```python
from build123d import *

# Parameters (mm, degrees)
BOSS_EXTRUDE1_DEPTH = 6.35
SKETCH2_R           = 2.5
CUT_EXTRUDE1_DEPTH  = 103.686827993


with BuildPart() as part:
    # Sketch1 → Boss-Extrude1 (new body)
    with BuildSketch(Plane(origin=(0, 0, 0), x_dir=(1, 0, 0), z_dir=(0, 1, 0))):
        with BuildLine():
            Line((5.368406408, 0), (44.345824206, 0))
            ThreePointArc((44.345824206, 0), (46.333684351, 0.753132838), (47.323462661, 2.63439197))
            Line((47.323462661, 2.63439197), (57.040137924, 81.77036144))
            ThreePointArc((57.040137924, 81.77036144), (55.05416359, 84.967329968), (51.507452969, 83.708145472))
            Line((51.507452969, 83.708145472), (2.813359907, 4.572176002))
            ThreePointArc((2.813359907, 4.572176002), (2.749577661, 1.536532885), (5.368406408, 0))
        make_face()
    extrude(amount=BOSS_EXTRUDE1_DEPTH)

    # Sketch2 → Cut-Extrude1 (cut, through all)
    with BuildSketch(Plane(origin=(0, 6.35, 0), x_dir=(1, 0, 0), z_dir=(0, 1, 0))):
        with Locations(Location((13.421016019, 7.5, 0), (0, 0, 270))):
            Circle(SKETCH2_R)
        with Locations(Location((46.29547273, 60.926439205, 0), (0, 0, 270))):
            Circle(SKETCH2_R)
        with Locations(Location((39.735530851, 7.5, 0), (0, 0, 270))):
            Circle(SKETCH2_R)
    extrude(amount=-CUT_EXTRUDE1_DEPTH, mode=Mode.SUBTRACT)


solid = part.part
```
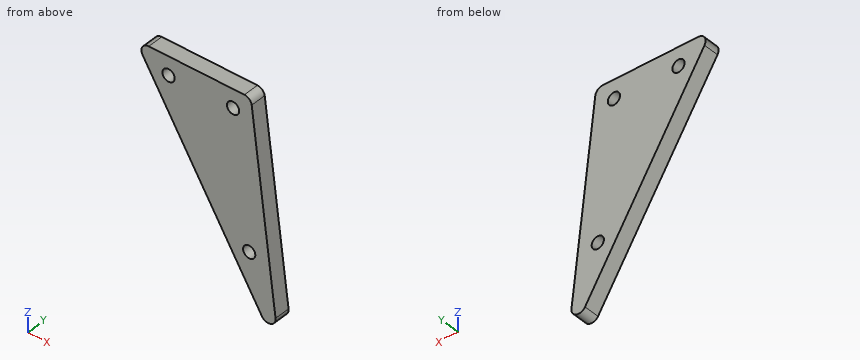
Design review of the part built by this model. Coordinates are the model's own, in mm. Give positions to 0.01 mm unless a question says otherwise; leave off trailing zeros. Loops run counter-clockwise (first coordinate to the right, second up) from the corner with the lowest first, then second, coordinate; pieces in that order, holes last. Notation, with made-up numbers: M -5,69.25 L 11,69.25 A33 ccw 11,105.25 Z; hole C 57,35 d2. An arc over 180 degrees is marked long. Return JSON: item names as keys, results as strings. Group by question number.
Item 1: We need section C-C (x = 30). Give the boundary of the cut face in (y, z).
Item 2: We need section B-B (y = 1.25). Give the boundary of the cut face in (x, z), and give its area (3 significant figures).
Item 3: For probe 1 along X at (y, z) = (1, -7.5); probe 2 along X at (y, z) = (3.25, -8.5); probe 3 along Z at (x, y) = (47, 4), list the stretches that pass through material, from the lowest coordinate up.
Item 4: We need section D-D (z = -22.5). Give the boundary of the cut face in (x, y).
Item 5: We need section A-A (z = -7). Give the boundary of the cut face in (x, y), and give its area (3 significant figures).
Item 6: Insertion check: pin 1 Ø2 at (y, z) = (3, -48) entering from +X; pin 2 Ø2 at (y, z) = (2.5, -34.5) entering from +X; pin 3 Ø2 at (y, z) = (1, -14.5) entering from -X; pin 4 Ø8 at (x, z) = (46.3, -60.93) entering from -Y. Each pin has a flat end and moves straight along its axis. Give the tip position at first contact, or say it passes through.
Output:
{
 "1": {"outline": "M 0,-48.75 L 6.35,-48.75 L 6.35,0 L 0,0 Z"},
 "2": {"outline": "M 2.81,-4.57 L 51.51,-83.71 A3 ccw 57.04,-81.77 L 47.32,-2.63 A3 ccw 44.35,0 L 5.37,0 A3 ccw Z; hole C 13.42,-7.5 d5; hole C 39.74,-7.5 d5; hole C 46.3,-60.93 d5", "area": "2,150 mm^2"},
 "3": {"probe 1": "x = 4.61 to 10.92, 15.92 to 37.24, 42.24 to 47.92", "probe 2": "x = 5.23 to 11.13, 15.71 to 37.44, 42.03 to 48.04", "probe 3": "z = -76.38 to -63.33, -58.53 to -1.6"},
 "4": {"outline": "M 13.84,0 L 49.76,0 L 49.76,6.35 L 13.84,6.35 Z"},
 "5": {"outline": "M 4.31,0 L 10.97,0 L 10.97,6.35 L 4.31,6.35 Z; M 15.87,0 L 37.29,0 L 37.29,6.35 L 15.87,6.35 Z; M 42.19,0 L 47.86,0 L 47.86,6.35 L 42.19,6.35 Z", "area": "214 mm^2"},
 "6": {"pin 1": "stops at x = 53.02", "pin 2": "stops at x = 51.36", "pin 3": "stops at x = 8.31", "pin 4": "stops at y = 0"}
}
